from build123d import *

# Parameters (mm, degrees)
BOSS_EXTRUDE1_DEPTH  = 4.7625
M4_CLEARANCE_HOLE1_D = 4.5


with BuildPart() as part:
    # Sketch1 → Boss-Extrude1 (new body)
    with BuildSketch(Plane.XY):
        with BuildLine():
            Line((166.110631803, -43.351929971), (117.238806396, -43.351929971))
            Line((117.238806396, -43.351929971), (117.238806396, -39.442229971))
            ThreePointArc((117.238806396, -39.442229971), (111.738806396, -33.942229971), (106.238806396, -39.442229971))
            Line((106.238806396, -39.442229971), (106.238806396, -43.351929971))
            Line((106.238806396, -43.351929971), (57.366980989, -43.351929971))
            Line((57.366980989, -43.351929971), (53.740076833, -39.725025815))
            ThreePointArc((53.740076833, -39.725025815), (45.96190224, -39.725025815), (45.96190224, -47.503200408))
            Line((45.96190224, -47.503200408), (49.588806396, -51.130104564))
            Line((49.588806396, -51.130104564), (49.588806396, -80.498755377))
            Line((49.588806396, -80.498755377), (45.96190224, -84.125659533))
            ThreePointArc((45.96190224, -84.125659533), (45.96190224, -91.903834126), (53.740076833, -91.903834126))
            Line((53.740076833, -91.903834126), (57.366980989, -88.276929971))
            Line((57.366980989, -88.276929971), (106.238806396, -88.276929971))
            Line((106.238806396, -88.276929971), (106.238806396, -92.186629971))
            ThreePointArc((106.238806396, -92.186629971), (111.738806396, -97.686629971), (117.238806396, -92.186629971))
            Line((117.238806396, -92.186629971), (117.238806396, -88.276929971))
            Line((117.238806396, -88.276929971), (166.110631803, -88.276929971))
            Line((166.110631803, -88.276929971), (169.737535958, -91.903834126))
            ThreePointArc((169.737535958, -91.903834126), (177.515710552, -91.903834126), (177.515710552, -84.125659533))
            Line((177.515710552, -84.125659533), (173.888806396, -80.498755377))
            Line((173.888806396, -80.498755377), (173.888806396, -51.130104564))
            Line((173.888806396, -51.130104564), (177.515710552, -47.503200408))
            ThreePointArc((177.515710552, -47.503200408), (177.515710552, -39.725025815), (169.737535958, -39.725025815))
            Line((169.737535958, -39.725025815), (166.110631803, -43.351929971))
        make_face()
    extrude(amount=BOSS_EXTRUDE1_DEPTH)

    # M4 Clearance Hole1 (through all)
    with Locations(Plane.XY.offset(4.7625)):
        with Locations((111.738806396, -39.442229971), (173.626623255, -43.614113111), (173.626623255, -88.01474683), (111.738806396, -92.186629971), (49.850989537, -88.01474683), (49.850989537, -43.614113111)):
            Hole(M4_CLEARANCE_HOLE1_D / 2)


solid = part.part
Source: CAD feature listing. Evaluate the final solid. Frame: model axes, mm. A direction names the side the tool comes from. Round coordinates to 2 decimals unless told otherwise and drop trailing zeros. Loops run counter-clockwise (first coordinate to the right, second up) from the corner with the lowest first, then second, coordinate; pieces in that order, holes last. Notation, with made-up numbers: (47, 45) -> (54, 45) arc R11 cw to (54, 66) -> close; hole circle Ø2 at (75.5, 65.5). An arc over 180 degrees is marked (long way). Answer as a JSON object with one key per item and string values. Group by question number.
Q1. Section query C-C (x = 95). Output: boundary loops of the cut face in (y, z).
Q2. Contact query for flat-ended pins moving along their axis: P1, Ø2.5, axis at x = 133, z = 1.5, coming from the -Y side; P2, Ø4, axis at x = 111.74, y = -39.44, coming from the +Z side; P3, Ø1.4, axis at y = -68, z = 2, coming from the -X side; P4, Ø2, axis at y = -56, z = 4, coming from the +X side. Output: stop coordinate, or through.
Q3. Mould query, pull axis X, two halves, no side actions, for faces 1 (the flat face through (55.528, -90.116, 2.348)), 2 (the flat face through (175.73, -82.34, 2.35)), 3 (the flat face through (47.75, -49.29, 2.35)). Classes: pulls with the +X half, pulls with the -X half, needs draft (parallel to the pull), parting line crosses it, or undercut.
Q4. Ray query, line 1 (X direction, y = -40.5, z = 4); line 2 (X direction, y = -86.5, z = 1.1); line 3 (X direction, y = -70.5, z = 0.6). Return the intervals inside material, ascending. Write a range as from..to.
Q5. Section query A-A (z = 1.2). State how many separate pieces and enclosed holes the cut face has, plus the area to 3 significant figures.
Q6. Access query for faces 4 (the flat face through (117.239, -41, 2)), 5 (the flat face through (47.8, -82.29, 2.35)), 6 (the cylindrical face through (46.05, -39.64, 2.35)), 7 (the flat face through (117.239, -90, 2)). Directions: +Z, -Z, +X, -X, +Y, -Y. A direction counts if a zero-diameter tool reaches every point of the face in a straight line with its end or side. Return the directions, or none.
Q7. Section query B-B (y = -73). Output: boundary loops of the cut face in (x, z), plus the area to 3 significant figures.
Completed:
{
 "1": {"outline": "(-88.28, 0) -> (-43.35, 0) -> (-43.35, 4.76) -> (-88.28, 4.76) -> close"},
 "2": {"P1": "y = -88.28", "P2": "through", "P3": "x = 49.59", "P4": "x = 173.89"},
 "3": {"face 1": "undercut", "face 2": "pulls with the +X half", "face 3": "pulls with the -X half"},
 "4": {"line 1": "45.32..54.52, 106.24..109.75, 113.72..117.24, 168.96..178.16", "line 2": "44.56..48.19, 51.51..171.96, 175.29..178.91", "line 3": "49.59..173.89"},
 "5": {"separate pieces": "1", "enclosed holes": "6", "area": "5,960 mm²"},
 "6": {"face 4": "+Z, -Z, +Y", "face 5": "+Z, -Z, -X", "face 6": "+Z, -Z", "face 7": "+Z, -Z, -Y"},
 "7": {"outline": "(49.59, 0) -> (173.89, 0) -> (173.89, 4.76) -> (49.59, 4.76) -> close", "area": "592 mm²"}
}
